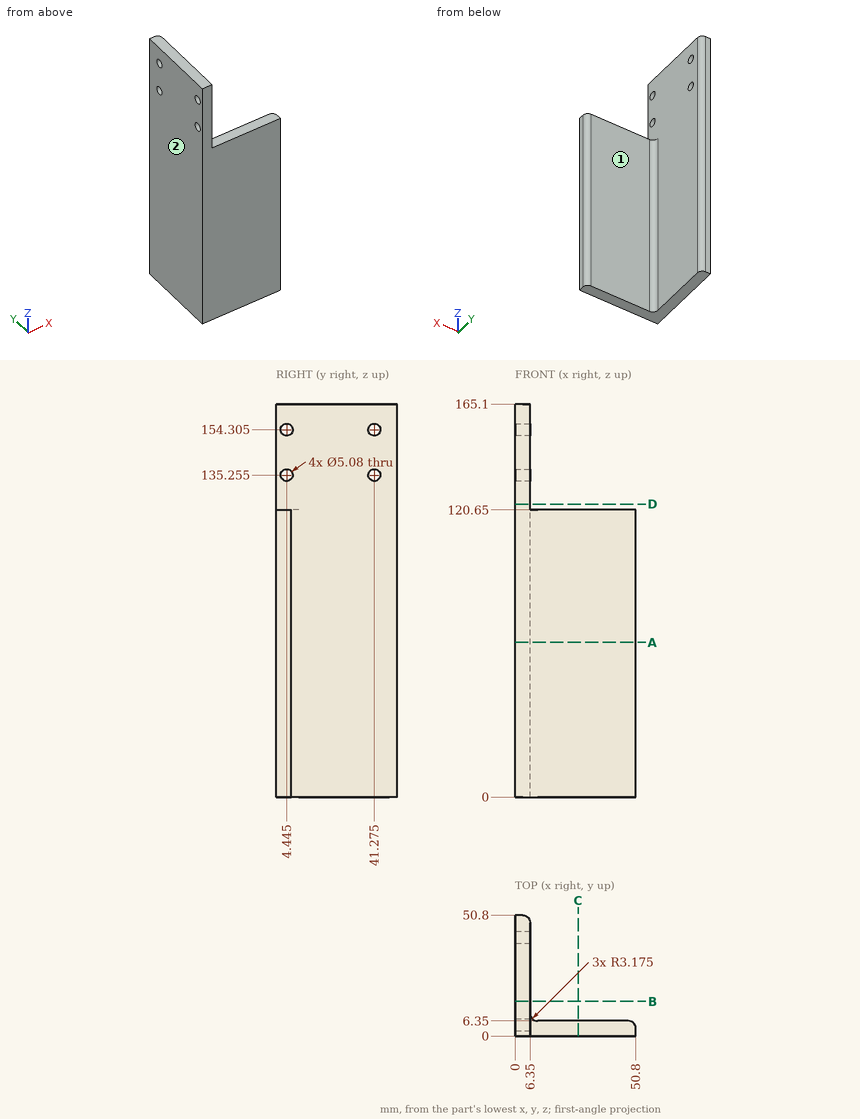
Print and shaded views of the part. All mm, measured from the part's lowest x, y and z. A direction names the side the tool comes from. Coordinates: 2 decimals unless noted, no trailing zeros. Order: outer loops, then holes, each group sorted by start corner. A loop starts at its lowest first (then second) coordinate and runs counter-clockwise, first axis right, second up. Notation, with made-up numbers: (64.5, -11.75) - (84.5, -11.75) arc R14 ccw to (84.5, 7.25) - close; hole circle Ø8 at (11.25, 25.25). An arc over 180 degrees is marked (long way). Put each result on its own line as item: value.
1. Saw through at B-B (y = 14.5). Write the cut outline in (x, z).
Answer sheet:
outline: (0, 0) - (6.35, 0) - (6.35, 165.1) - (0, 165.1) - close
2. Drop flat-ended pins along their axis: P1, Ø8, axis at y = 4.445, z = 154.305, coming from the +X side; P2, Ø5, axis at x = 32, z = 53, coming from the +Y side; P3, Ø3, axis at y = 41.275, z = 154.305, coming from the +X side; P4, Ø3, axis at x = 31.5, y = 4, coming from the +Z side. Give the stop position or say it passes through.
Answer sheet:
P1: stops at x = 6.35
P2: stops at y = 6.35
P3: passes through
P4: stops at z = 120.65
3. Saw through at C-C (x = 26.5). Write the cut outline in (y, z), and give its area (3 significant figures).
Answer sheet:
outline: (0, 0) - (6.35, 0) - (6.35, 120.65) - (0, 120.65) - close
area: 766 mm^2
4. Probe line 1 along X through (y, z) = (48, 110); line 2 along X through (y, z) = (45, 25). List the from-to ranges inside material, lowest first. Write a range as [from, to].
Answer sheet:
line 1: x = [0, 6.33]
line 2: x = [0, 6.35]
5. Tool access for the marked faces 1 and 2: list every direction of +Z, -Z, +X, -X, +Y, -Y with a clear straight run to the whole face (end or side of a thin tool).
Answer sheet:
face 1: +Z, -Z, +X, +Y
face 2: +Z, -Z, -X, +Y, -Y
6. Saw through at A-A (z = 65). Write the cut outline in (x, y) (3 decimals), and give its area (3 significant figures).
Answer sheet:
outline: (0, 0) - (50.8, 0) - (50.8, 3.175) arc R3.175 ccw to (47.625, 6.35) - (9.525, 6.35) arc R3.175 cw to (6.35, 9.525) - (6.35, 47.625) arc R3.175 ccw to (3.175, 50.8) - (0, 50.8) - close
area: 603 mm^2
7. Saw through at D-D (z = 123). Write the cut outline in (x, y) (3 decimals).
Answer sheet:
outline: (0, 0) - (6.35, 0) - (6.35, 47.625) arc R3.175 ccw to (3.175, 50.8) - (0, 50.8) - close
